Verification items for the finished model (mm, model axes). Face numbers are marked on the shaded views. A direction names the side the tool comes from. Coordinates: 2 decimals unless noted, no trailing zeros. Write each loop counter-clockwise with the first axis right and the second up, starting at its lowest first coordinate (ties: lowest second). Pieces come first, ordered by that corner, then holes. Notation, with made-up numbers: (-1.75, 30.5) -> (2.25, 30.5) arc R34 ccw to (2.25, 60.5) -> close; hole circle Ø3 at (-8, 45). An arc over 180 degrees is marked (long way). Write item = value, one per line. Start each with the question number.
(1) Section check A-A (y = 0). Record the cut outline in (x, z).
(2) Gauge pin test, flat ends, axial feed: pin 1 Ø2 at (x, z) = (-16, 7) entering from -Y; pin 2 Ø1 at (x, z) = (26.5, 13) entering from +Y; pin 3 Ø12 at (x, z) = (27.5, 7.5) entering from -Y. Record the tip position at first contact, or that the pin passes through.
(3) Set-up check for the marked faces 1 and 2: record each of +Z, -Z, +X, -X, +Y, -Y from which the full face is reachable in a straight line by a thin tool's end or side.
(4) Mould release check, pull along X, two halves, no side actions. Record for the marked faces 3, 4 and 5: released by +X, released by -X, zero draft, split by the parting line, or undercut.
(5) Material ranges on probe 1 along Z at (x, y) = (21.5, -39); probe 2 along Y at (x, z) = (0, 18.5); probe 3 along X at (y, z) = (10, 12.25), recorded low to high. Write a range as [from, to].
(6) Section check C-C (z = 10.5). Record the cut outline in (x, y).
```python
from build123d import *

# Parameters (mm, degrees)
SKETCH1_R           = 45
BOSS_EXTRUDE1_DEPTH = 9
SKETCH2_R           = 32.5
BOSS_EXTRUDE4_DEPTH = 7
SKETCH4_R           = 45
BOSS_EXTRUDE5_DEPTH = 9
SKETCH5_R           = 27.5
CUT_EXTRUDE1_DEPTH  = 25


with BuildPart() as part:
    # Sketch1 → Boss-Extrude1 (new body)
    with BuildSketch(Plane.XY):
        Circle(SKETCH1_R)
    extrude(amount=BOSS_EXTRUDE1_DEPTH)

    # Sketch2 → Boss-Extrude4 (add)
    with BuildSketch(Plane.XY.offset(9)):
        Circle(SKETCH2_R)
    extrude(amount=BOSS_EXTRUDE4_DEPTH)

    # Sketch4 → Boss-Extrude5 (add)
    with BuildSketch(Plane.XY.offset(16)):
        Circle(SKETCH4_R)
    extrude(amount=BOSS_EXTRUDE5_DEPTH)

    # Sketch5 → Cut-Extrude1 (cut)
    with BuildSketch(Plane.XY.offset(25)):
        Circle(SKETCH5_R)
    extrude(amount=-CUT_EXTRUDE1_DEPTH, mode=Mode.SUBTRACT)


solid = part.part
```
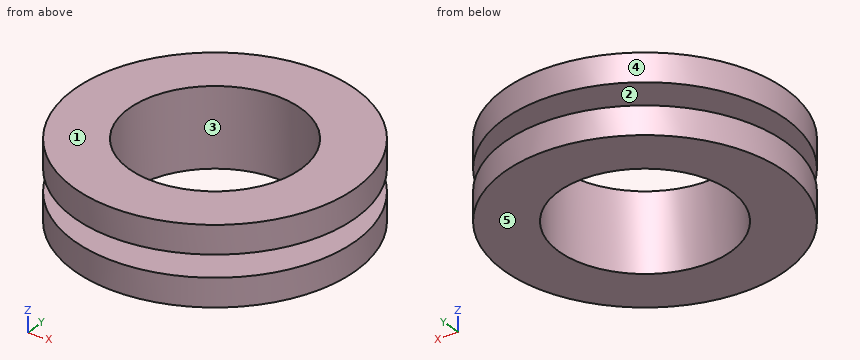
Response:
q1.outline = (-45, 0) -> (-27.5, 0) -> (-27.5, 25) -> (-45, 25) -> (-45, 16) -> (-32.5, 16) -> (-32.5, 9) -> (-45, 9) -> close; (27.5, 0) -> (45, 0) -> (45, 9) -> (32.5, 9) -> (32.5, 16) -> (45, 16) -> (45, 25) -> (27.5, 25) -> close
q2.pin_1 = -42.43
q2.pin_2 = 19.5
q2.pin_3 = -39.53
q3.face_1 = +Z, +X, -X, +Y, -Y
q3.face_2 = none
q4.face_3 = undercut
q4.face_4 = split by the parting line
q4.face_5 = zero draft
q5.probe_1 = [0, 9], [16, 25]
q5.probe_2 = [-45, -27.5], [27.5, 45]
q5.probe_3 = [-30.92, -25.62], [25.62, 30.92]
q6.outline = circle Ø65 at (0, 0); hole circle Ø55 at (0, 0)
